Part model, mm, in its own coordinate system. A direction names the side the tool comes from. Coordinates: 2 decimals unless noted, no trailing zeros. Loops run counter-clockwise (first coordinate to the right, second up) from the corner with the lowest first, then second, coordinate; pieces in that order, holes last. Notation, with made-up numbers: (75.5, 59.5) - (101.5, 59.5) arc R13 cw to (101.5, 66.5) - close; hole circle Ø8 at (40, 64.5). An arc over 180 degrees is marked (long way). Use a Markdown table: item, result. Add a question column.
1. Drop flat-ended pins along their axis: pin 1 (2 mm diameter, centred on x = 138, y = 15.5, fed in from +Z); pin 2 (5 mm diameter, centred on x = 140, z = 25.5, fed in from +Y); pin 3 (10 mm diameter, centred on y = 15, z = 24.95, fed in from -X). Give the stop position or say it passes through.
2. 3-axis set-ups, long thin cutter, end or side, ignore diameter. For faces 4 (the flat face through (141, 25.8, 0)), 5 (the flat face through (140, 15, 30.1)), 6 (the flat face through (144, 24.8, -7)): which of +Z, -Z, +X, -X, +Y, -Y reach the whole face in a straight line?
3. Pull direction Y, two halves, no side cores. Call faces 1 (the cylindrical face through (139.84, 25.23, 30.5)), 2 (the cylindrical face through (148.8, 13.1, 27.4)), 3 (the flat face through (148, 15, -32.5)): pulls with the +Y half, pulls with the -Y half, needs draft (parallel to the pull), parting line crosses it, or undercut.
4. Band-saw the part on B-B, the plane x = 150.75. Give the cut face in (y, z), plus the area to 3 significant figures.
5. Band-saw the part on A-A, the plane y = 22.5. Give the cut face in (x, z) (3 decimals).
6. Wall check: probe 1 along Z at (x, y) = (145.5, 21.5); probe 2 along Z at (x, y) = (145, 15.5); probe 3 along Z at (x, y) = (137.75, 16.5). Give the ranges that are in metal, low to high. Write a range as [from, to].
7. Band-saw the part on D-D, the plane y = 15. Count the separate pieces of the cut face and the enclosed holes in it, plus the area to 3 significant figures.
8. Band-saw the part on C-C, the plane z = 7.3. Give the cut face in (x, y), plus the area to 3 significant figures.
from build123d import *

# Parameters (mm, degrees)
BOSS_EXTRUDE1_DEPTH = 30
SKETCH2_W           = 62.2
SKETCH2_H           = 21.6
BOSS_EXTRUDE2_DEPTH = 17
SKETCH2_6_R         = 2.1
SKETCH2_6_R_2       = 3.1
SKETCH2_6_W         = 13.4
SKETCH2_6_H         = 19.6
CUT_EXTRUDE3_DEPTH  = 17
CUT_EXTRUDE5_START  = -7
SKETCH2_8_W         = 7.5
SKETCH2_8_H         = 7.5
SKETCH2_8_R         = 2.1
SKETCH2_8_W_2       = 10.3
SKETCH2_8_H_2       = 11
SKETCH2_8_R_2       = 3.1
CUT_EXTRUDE5_DEPTH  = 10
FILLET1_R           = 2


with BuildPart() as part:
    # Sketch1 → Boss-Extrude1 (new body)
    with BuildSketch(Plane(origin=(0, 0, 0), x_dir=(1, 0, 0), z_dir=(0, 1, 0))):
        with BuildLine():
            Line((152.287802769, 32.5), (143.787802769, 32.5))
            ThreePointArc((143.787802769, 32.5), (146.505394389, 16.350891105), (147.415, 0))
            ThreePointArc((147.415, 0), (146.505394389, -16.350891105), (143.787802769, -32.5))
            Line((143.787802769, -32.5), (152.287802769, -32.5))
            Line((152.287802769, -32.5), (152.287802769, 32.5))
        make_face()
    extrude(amount=BOSS_EXTRUDE1_DEPTH)

    # Sketch2 → Boss-Extrude2 (add)
    with BuildSketch(Plane(origin=(152.287802769, 0, 0), x_dir=(0, 0, -1), z_dir=(1, 0, 0))):
        with Locations((0, 15)):
            Rectangle(SKETCH2_W, SKETCH2_H)
    extrude(amount=-BOSS_EXTRUDE2_DEPTH)

    # Sketch2<6> → Cut-Extrude3 (cut)
    with BuildSketch(Plane(origin=(152.287802769, 0, 0), x_dir=(0, 0, -1), z_dir=(1, 0, 0))):
        with Locations((-7.3, 15)):
            Circle(SKETCH2_6_R)
        with Locations((-24.95, 15)):
            Circle(SKETCH2_6_R_2)
        with Locations((23.4, 15)):
            Rectangle(SKETCH2_6_W, SKETCH2_6_H)
        with Locations((6.65, 15)):
            Rectangle(SKETCH2_6_W, SKETCH2_6_H)
    extrude(amount=-CUT_EXTRUDE3_DEPTH, mode=Mode.SUBTRACT)

    # Sketch2<8> → Cut-Extrude5 (cut)
    with BuildSketch(Plane(origin=(152.287802769, 0, 0), x_dir=(0, 0, -1), z_dir=(1, 0, 0)).offset(CUT_EXTRUDE5_START)):
        with Locations((-7.3, 15)):
            Rectangle(SKETCH2_8_W, SKETCH2_8_H)
        with Locations((-7.3, 15)):
            Circle(SKETCH2_8_R, mode=Mode.SUBTRACT)
        with Locations((-24.95, 15)):
            Rectangle(SKETCH2_8_W_2, SKETCH2_8_H_2)
        with Locations((-24.95, 15)):
            Circle(SKETCH2_8_R_2, mode=Mode.SUBTRACT)
    extrude(amount=-CUT_EXTRUDE5_DEPTH, mode=Mode.SUBTRACT)

    # Fillet1
    fillet1_edges = [part.edges().sort_by_distance(p)[0] for p in [
        (139.692447908, 25.8, 31.1),
        (139.692447908, 25.8, -31.1),
        (139.692447908, 4.2, -31.1),
        (139.692447908, 4.2, 31.1),
    ]]
    fillet(fillet1_edges, radius=FILLET1_R)


solid = part.part
Geometry check:
| question | item | result |
|---|---|---|
| 1 | pin 1 | stops at z = 31.1 |
| 1 | pin 2 | stops at y = 25.8 |
| 1 | pin 3 | stops at x = 145.29 |
| 2 | face 4 | -X, +Y |
| 2 | face 5 | -X |
| 2 | face 6 | +X, -X |
| 3 | face 1 | pulls with the +Y half |
| 3 | face 2 | undercut |
| 3 | face 3 | needs draft |
| 4 | outline | (0, -32.5) - (30, -32.5) - (30, 32.5) - (0, 32.5) - close; hole (5.2, -30.1) - (24.8, -30.1) - (24.8, -16.7) - (5.2, -16.7) - close; hole (5.2, -13.35) - (24.8, -13.35) - (24.8, 0.05) - (5.2, 0.05) - close; hole circle Ø6.2 at (15, 24.95); hole circle Ø4.2 at (15, 7.3) |
| 4 | area | 1,380 mm^2 |
| 5 | outline | (135.288, -31.1) - (144.097, -31.1) arc R147.415 cw to (143.788, -32.5) - (152.288, -32.5) - (152.288, -30.1) - (135.288, -30.1) - close; (135.288, -16.7) - (152.288, -16.7) - (152.288, -13.35) - (135.288, -13.35) - close; (135.288, 0.05) - (152.288, 0.05) - (152.288, 32.5) - (143.788, 32.5) arc R147.415 cw to (144.097, 31.1) - (135.288, 31.1) - close |
| 6 | probe 1 | z = [-32.5, -30.1], [-16.7, -13.35], [0.05, 32.5] |
| 6 | probe 2 | z = [-32.5, -30.1], [-16.7, -13.35], [0.05, 3.55], [11.05, 19.8], [30.1, 32.5] |
| 6 | probe 3 | z = [-31.1, -30.1], [-16.7, -13.35], [0.05, 3.55], [11.05, 19.8], [30.1, 31.1] |
| 7 | separate pieces | 5 |
| 7 | enclosed holes | 0 |
| 7 | area | 374 mm^2 |
| 8 | outline | (135.29, 4.2) - (147.23, 4.2) - (147.23, 0) - (152.29, 0) - (152.29, 12.9) - (145.29, 12.9) - (145.29, 11.25) - (135.29, 11.25) - close; (135.29, 18.75) - (145.29, 18.75) - (145.29, 17.1) - (152.29, 17.1) - (152.29, 30) - (147.23, 30) - (147.23, 25.8) - (135.29, 25.8) - close |
| 8 | area | 305 mm^2 |
